Answer from the drawing. Dimensions are ordinates in mm from the lowest x, y and z of the part. A direction names the side the tool comes from. Give positions to 0.01 mm unless a question says otherwise; leave off trailing zeros. Write each loop counter-clockwise with the first axis right and the second up, starting at its lowest first coordinate (ties: lowest second). Pieces come first, ordered by that corner, then holes. Notation, with made-up numbers: M 6,-30 L 62,-30 A21 cw 62,0 Z; hole C 51,-11.5 d1. An arc over 180 degrees is marked long. Put each result on its own line as item: value.
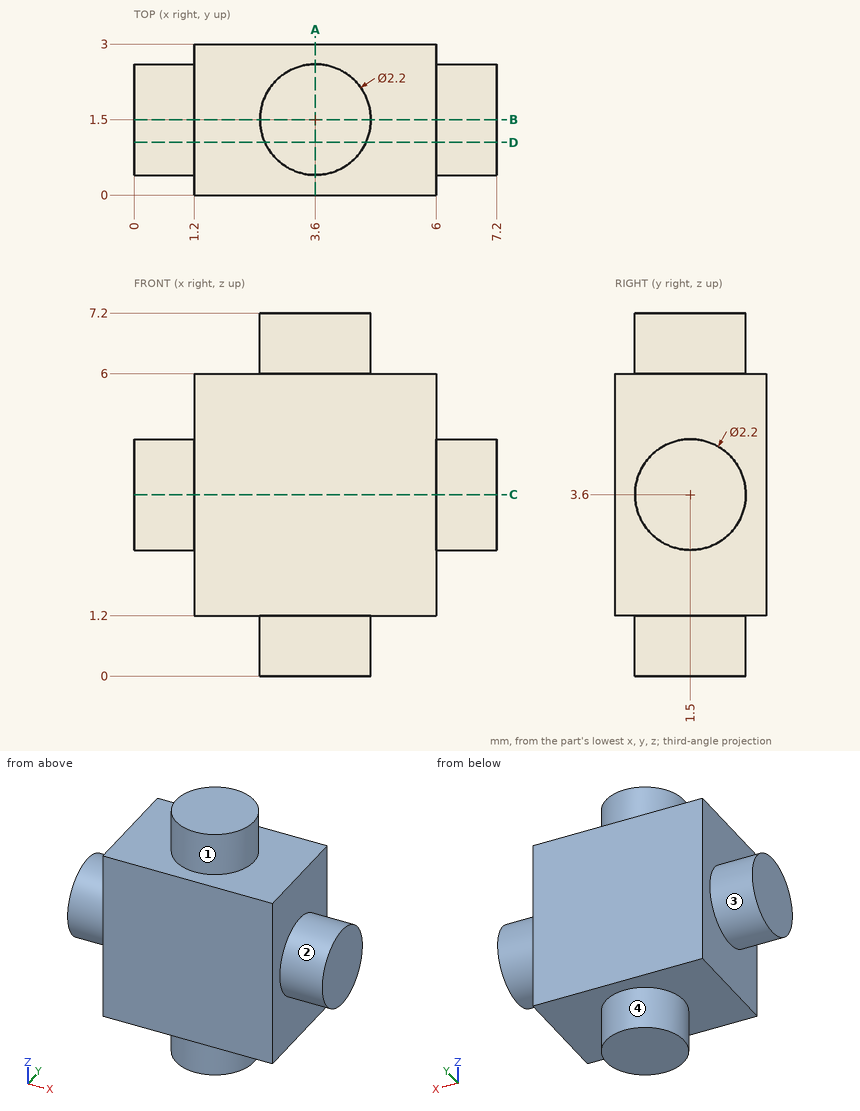
(1) Section D-D on y = 1.05 is taken. Determine the outline of the cut face in (x, z), and give its area (3 significant figures).
Result:
outline: M 0,2.6 L 1.2,2.6 L 1.2,1.2 L 2.6,1.2 L 2.6,0 L 4.6,0 L 4.6,1.2 L 6,1.2 L 6,2.6 L 7.2,2.6 L 7.2,4.6 L 6,4.6 L 6,6 L 4.6,6 L 4.6,7.2 L 2.6,7.2 L 2.6,6 L 1.2,6 L 1.2,4.6 L 0,4.6 Z
area: 32.7 mm²
(2) Section C-C on z = 3.6 is taken. Determine the outline of the cut face in (x, y), and give its area (3 significant figures).
Result:
outline: M 0,0.4 L 1.2,0.4 L 1.2,0 L 6,0 L 6,0.4 L 7.2,0.4 L 7.2,2.6 L 6,2.6 L 6,3 L 1.2,3 L 1.2,2.6 L 0,2.6 Z
area: 19.7 mm²
(3) Which of the six approach directions +Z, -Z, +X, -X, +Y, -Y give full straight-line access (tool end or side, diameter ignored) to the marked faces 1, 2, 3 and 4?
Result:
face 1: +Z
face 2: +X
face 3: -X
face 4: -Z
(4) Section A-A on x = 3.6 is taken. Determine the outline of the cut face in (y, z), and give its area (3 significant figures).
Result:
outline: M 0,1.2 L 0.4,1.2 L 0.4,0 L 2.6,0 L 2.6,1.2 L 3,1.2 L 3,6 L 2.6,6 L 2.6,7.2 L 0.4,7.2 L 0.4,6 L 0,6 Z
area: 19.7 mm²
(5) Straight lines are drawn through the part: line 1 along Z through (x, y) = (1.25, 0.4); line 2 along Y through (x, z) = (3, 0.75). For each, find the intervals that lie inside material, in ascending order. Write a range as from..to.
Result:
line 1: z = 1.2..6
line 2: y = 0.58..2.42
(6) Section B-B on y = 1.5 is taken. Determine the outline of the cut face in (x, z).
Result:
outline: M 0,2.5 L 1.2,2.5 L 1.2,1.2 L 2.5,1.2 L 2.5,0 L 4.7,0 L 4.7,1.2 L 6,1.2 L 6,2.5 L 7.2,2.5 L 7.2,4.7 L 6,4.7 L 6,6 L 4.7,6 L 4.7,7.2 L 2.5,7.2 L 2.5,6 L 1.2,6 L 1.2,4.7 L 0,4.7 Z
